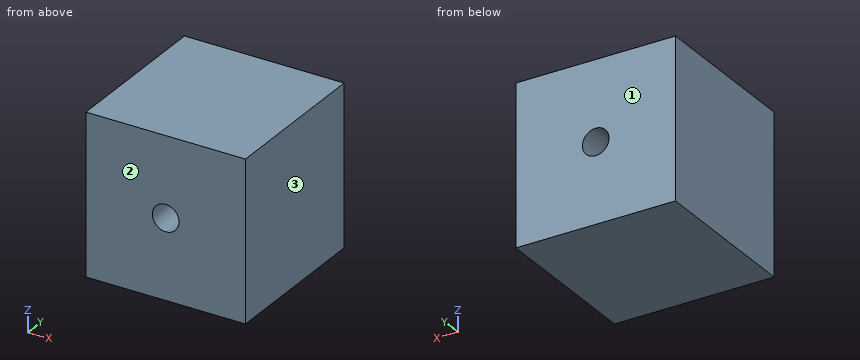
```python
from build123d import *

# Parameters (mm, degrees)
F0_W     = 152.4
F0_H     = 152.4
F0_R     = 12.7
F1_DEPTH = 152.4
F2_DEPTH = 152.4


with BuildPart() as f1:
    # F0 (on Front) → F1 (new body)
    with BuildSketch(Plane.XZ):
        Rectangle(F0_W, F0_H)
        Circle(F0_R, mode=Mode.SUBTRACT)
    extrude(amount=F1_DEPTH)

    # F0 (on Front) → F2 (cut)
    with BuildSketch(Plane.XZ):
        Rectangle(F0_W, F0_H)
        Circle(F0_R, mode=Mode.SUBTRACT)
    extrude(amount=-F2_DEPTH, mode=Mode.SUBTRACT)


solid = f1.part
```
Here's how the part is built. I have some questions about the finished solid (model axes, mm). Face numbers are marked on the shaded views. Round coordinates to 2 decimals unless told otherwise and drop trailing zeros. Write each loop counter-clockwise with the first axis right and the second up, starting at its lowest first coordinate (ties: lowest second). Pieces come first, ordered by that corner, then holes.
Q1. If we section it at C-C on y = -91.5: Write out the boundary of the cut face in (x, z), plus the area to 3 significant figures.
Q2. If we section it at A-A on x = 0: Write out the boundary of the cut face in (y, z), plus the area to 3 significant figures.
Q3. Please list where these lines run through material, in increasing order: probe 1 along Z at (x, y) = (0, -33); probe 2 along Z at (x, y) = (2, -36.5); probe 3 along X at (y, z) = (-10, 10.5).
Q4. If we section it at B-B on z = 0: Write out the boundary of the cut face in (x, y), plus the area to 3 significant figures.
Q5. If we mould it in two halves opening along Y, with no side actions, what happens to the marked faces 1, 2 and 3? For each: +Y half, -Y half, draft (parallel to the pull), parting line (faces both ways), or undercut.
Answer below:
1. outline: (-76.2, -76.2) - (76.2, -76.2) - (76.2, 76.2) - (-76.2, 76.2) - close; hole circle Ø25.4 at (0, 0)
1. area: 22,700 mm2
2. outline: (-152.4, -76.2) - (0, -76.2) - (0, -12.7) - (-152.4, -12.7) - close; (-152.4, 12.7) - (0, 12.7) - (0, 76.2) - (-152.4, 76.2) - close
2. area: 19,400 mm2
3. probe 1: z = -76.2 to -12.7, 12.7 to 76.2
3. probe 2: z = -76.2 to -12.54, 12.54 to 76.2
3. probe 3: x = -76.2 to -7.14, 7.14 to 76.2
4. outline: (-76.2, -152.4) - (-12.7, -152.4) - (-12.7, 0) - (-76.2, 0) - close; (12.7, -152.4) - (76.2, -152.4) - (76.2, 0) - (12.7, 0) - close
4. area: 19,400 mm2
5. face 1: +Y half
5. face 2: -Y half
5. face 3: draft
